Could you check a few things on this model? Use its own coordinates, in mm. A direction names the side the tool comes from. Round coordinates to 2 decimals unless told otherwise and drop trailing zeros. Loops run counter-clockwise (first coordinate to the right, second up) from the corner with the lowest first, then second, coordinate; pieces in that order, holes last. Notation, with made-up numbers: (87, 77) -> (127, 77) arc R24 cw to (127, 116) -> close; hole circle Ø6 at (-30.5, 54). An arc over 180 degrees is marked (long way). One line per item, written item: value.
```python
from build123d import *

# Parameters (mm, degrees)
ESQUISSE1_W        = 45
ESQUISSE1_H        = 45
ESQUISSE1_R        = 16.25
BOSS_EXTRU_1_DEPTH = 5
ESQUISSE2_R        = 18.75
ESQUISSE2_R_2      = 16.25
BOSS_EXTRU_2_DEPTH = 20
ESQUISSE3_W        = 4.8
ESQUISSE3_H        = 3.8
BOSS_EXTRU_3_DEPTH = 3


with BuildPart() as part:
    # Esquisse1 → Boss.-Extru.1 (new body)
    with BuildSketch(Plane.XY):
        Rectangle(ESQUISSE1_W, ESQUISSE1_H)
        Circle(ESQUISSE1_R, mode=Mode.SUBTRACT)
    extrude(amount=BOSS_EXTRU_1_DEPTH)

    # Esquisse2 → Boss.-Extru.2 (add)
    with BuildSketch(Plane.XY.offset(5)):
        Circle(ESQUISSE2_R)
        Circle(ESQUISSE2_R_2, mode=Mode.SUBTRACT)
    extrude(amount=BOSS_EXTRU_2_DEPTH)

    # Esquisse3 → Boss.-Extru.3 (add)
    with BuildSketch(Plane(origin=(0, 0, 0), x_dir=(-1, 0, 0), z_dir=(0, 0, -1))):
        with Locations((16.4, 16.9)):
            Rectangle(ESQUISSE3_W, ESQUISSE3_H)
        with Locations((-16.4, 16.9)):
            Rectangle(ESQUISSE3_W, ESQUISSE3_H)
        with Locations((-16.4, -16.9)):
            Rectangle(ESQUISSE3_W, ESQUISSE3_H)
        with Locations((16.4, -16.9)):
            Rectangle(ESQUISSE3_W, ESQUISSE3_H)
    extrude(amount=BOSS_EXTRU_3_DEPTH)


solid = part.part
```
Item 1: If we section it at D-D on y = 19.5: List the corners of the cut face in (x, z) for me.
Output:
outline: (-22.5, 0) -> (22.5, 0) -> (22.5, 5) -> (-22.5, 5) -> close
Item 2: If we section it at A-A on y = 0: List the corners of the cut face in (x, z) for me.
Output:
outline: (-22.5, 0) -> (-16.25, 0) -> (-16.25, 25) -> (-18.75, 25) -> (-18.75, 5) -> (-22.5, 5) -> close; (16.25, 0) -> (22.5, 0) -> (22.5, 5) -> (18.75, 5) -> (18.75, 25) -> (16.25, 25) -> close
Item 3: If we mould it in two halves opening along Y, with no side actions, what happens to faces 4 (the face through (16, -18.8, -1)), 5 (the face through (18.8, -17, -1)), 6 (the face through (16, -15, -1)), 7 (the face through (0, 22.5, 2))? For each: released by +Y, released by -Y, zero draft, split by the parting line, or undercut.
Output:
face 4: released by -Y
face 5: zero draft
face 6: undercut
face 7: released by +Y
Item 4: For faces 1 (the face through (16, 18.8, -1)), 2 (the face through (-14, -17, -1)), 3 (the face through (18.8, 17, -1)), which set-ups out of +Z, -Z, +X, -X, +Y, -Y let a thin tool reach every point of the face, with its end or its side?
Output:
face 1: -Z, +X, -X, +Y
face 2: -Z, +Y, -Y
face 3: -Z, +X, +Y, -Y
Item 5: If we section it at C-C on z = 9.25: List the corners of the cut face in (x, y) for me.
Output:
outline: circle Ø37.5 at (0, 0); hole circle Ø32.5 at (0, 0)
Item 6: I need wall thicknesses on line 1 (Y direction, x = 0, z = 15); line 2 (Y direction, x = 10, z = 10); line 3 (Z direction, x = -5, y = 15.5). Which ranges of each line are inside material? Lowest first, please. Write a range as from..to.
Output:
line 1: y = -18.75..-16.25, 16.25..18.75
line 2: y = -15.86..-12.81, 12.81..15.86
line 3: z = 0..25
Item 7: Will these pins go through, and if not, where does the flat tip stop? pin 1 Ø0.9 at (x, z) = (-16.5, -1.5) entering from +Y; pin 2 Ø6 at (y, z) = (-7, 20) entering from -X; pin 3 Ø5 at (x, z) = (4, 8.5) entering from -Y.
Output:
pin 1: stops at y = 18.8
pin 2: stops at x = -18.32
pin 3: stops at y = -18.69
